Verification items for the finished model (mm, model axes). Round coordinates to 2 decimals unless told otherwise and drop trailing zeros. Write each loop counter-clockwise with the first axis right and the second up, starting at its lowest first coordinate (ties: lowest second). Pieces come first, ordered by that corner, then holes. Notation, with made-up numbers: M 9,22 L 61,22 A22 ccw 61,34 Z; hole C 56.25,67.25 d3. An arc over 180 degrees is marked long. Answer in a Markdown table with one row per item. Add a question column.
1. Sectioned sample at B-B on x = 18.5. Record the cut outline in (y, z) (3 decimals), plus the area to 3 significant figures.
2. Sectioned sample at D-D on z = -62.5. Record the cut outline in (x, y) (3 decimals).
3. Sectioned sample at C-C on x = 30. Record the cut outline in (y, z) (3 decimals).
4. Go/stop test with flat-tipped pins: pin 1 Ø3.5 at (x, z) = (37.11, -55.54) entering from +Y; pin 2 Ø1.9 at (y, z) = (-1.5, -24.5) entering from -X; pin 3 Ø2 at (x, y) = (4.5, 2) entering from -Z; pin 4 Ø4 at (x, z) = (65.52, 13.03) entering from -Y (3 decimals). Record where each tip stops, or that it passes through.
5. Sectioned sample at A-A on z = -3.5. Record the cut outline in (x, y) (3 decimals).
6. Material ranges on probe 1 along Y at (x, z) = (0, -70) (3 decimals); probe 2 along Z at (x, y) = (44.5, 0); probe 3 along Z at (x, y) = (42, 2.25), recorded low to high.
```python
from build123d import *

# Parameters (mm, degrees)
SKETCH1_R                                       = 7.5
BOSS_EXTRUDE1_DEPTH                             = 3.175
CIRPATTERN1_COUNT                               = 3
CIRPATTERN1_ANGLE                               = 135
M3_CLEARANCE_HOLE1_D                            = 3.2
M3_CLEARANCE_HOLE1_DEPTH                        = 15
CSK_FOR_M3_FLAT_HEAD_MACHINE_SCREW1_D           = 3.2
CSK_FOR_M3_FLAT_HEAD_MACHINE_SCREW1_CSINK_D     = 6.3
CSK_FOR_M3_FLAT_HEAD_MACHINE_SCREW1_CSINK_ANGLE = 90
CUT_EXTRUDE1_REACH                              = 107.268
FILLET1_R                                       = 3.175
CUT_EXTRUDE2_REACH                              = 107.268
SKETCH11_W                                      = 9.65
SKETCH11_H                                      = 32.732103654
F_1_4_CLEARANCE_HOLE1_D                         = 6.7564


with BuildPart() as part:
    # Sketch1 → Boss-Extrude1 (new, symmetric)
    with BuildSketch(Plane(origin=(0, 0, 0), x_dir=(1, 0, 0), z_dir=(0, 1, 0))):
        with BuildLine():
            Line((-13.85, 35), (-7.5, 35))
            Line((-7.5, 35), (-7.5, 15))
            Line((-7.5, 15), (-16.770509831, 15))
            ThreePointArc((-16.770509831, 15), (-18.002512666, -13.496649128), (9.696699141, -20.303300859))
            Line((9.696699141, -20.303300859), (46.966384428, -57.572986146))
            ThreePointArc((46.966384428, -57.572986146), (68.644249266, 28.433379025), (-7.5, 73.920497834))
            Line((-7.5, 73.920497834), (-7.5, 45))
            Line((-7.5, 45), (-13.85, 45))
            Line((-13.85, 45), (-13.85, 35))
        make_face()
        with Locations(Location((0, 0, 0), (0, 0, 270))):
            Circle(SKETCH1_R, mode=Mode.SUBTRACT)
        with BuildLine():
            Line((20.303300859, -9.696699141), (46.898012061, -36.291410343))
            ThreePointArc((46.898012061, -36.291410343), (58.160567128, -11.568856096), (57.216234934, 15.581798996))
            Line((57.216234934, 15.581798996), (22.468570216, 1.188845008))
            ThreePointArc((22.468570216, 1.188845008), (22.067668809, -4.389532245), (20.303300859, -9.696699141))
        make_face(mode=Mode.SUBTRACT)
        with BuildLine():
            Line((7.5, 15), (7.5, 35))
            Line((7.5, 35), (13.85, 35))
            Line((13.85, 35), (13.85, 45))
            Line((13.85, 45), (7.5, 45))
            Line((7.5, 45), (7.5, 58.823804705))
            ThreePointArc((7.5, 58.823804705), (32.945314818, 49.30614801), (51.475983449, 29.439991983))
            Line((51.475983449, 29.439991983), (16.72831873, 15.047037996))
            Line((16.72831873, 15.047037996), (16.614758962, 15))
            Line((16.614758962, 15), (7.5, 15))
        make_face(mode=Mode.SUBTRACT)
    extrude(amount=BOSS_EXTRUDE1_DEPTH, both=True)

    # Sketch5 → M2.2x0.45 Tapped Hole1 (revolve, cut)
    with BuildSketch(Plane(origin=(0, 0, -74.3), x_dir=(0, 1, 0), z_dir=(1, 0, 0))):
        Polygon((0, 0), (0, 10.525753042), (0.875, 10), (0.875, 0), align=None)
    m2_2x0_45_tapped_hole1 = revolve(axis=Axis((0, 0, -80.65), (0, 0, 1)), mode=Mode.SUBTRACT)

    # CirPattern1: M2.2x0.45 Tapped Hole1 ×3 about axis
    cirpattern1_axis = Axis((0, 3.175, 0), (0, -1, 0))
    for i in range(1, CIRPATTERN1_COUNT):
        add(m2_2x0_45_tapped_hole1.rotate(cirpattern1_axis, i * CIRPATTERN1_ANGLE / (CIRPATTERN1_COUNT - 1)), mode=Mode.SUBTRACT)

    # M3 Clearance Hole1
    with Locations(Plane.ZY.offset(7.5)):
        with Locations((-25, 0)):
            Hole(M3_CLEARANCE_HOLE1_D / 2, depth=M3_CLEARANCE_HOLE1_DEPTH)

    # CSK for M3 Flat Head Machine Screw1 (through all)
    with Locations(Plane(origin=(0, 3.175, 0), x_dir=(1, 0, 0), z_dir=(0, 1, 0))):
        with Locations((65.516456731, -13.032033511), (37.112091566, 55.542170102)):
            CounterSinkHole(CSK_FOR_M3_FLAT_HEAD_MACHINE_SCREW1_D / 2, CSK_FOR_M3_FLAT_HEAD_MACHINE_SCREW1_CSINK_D / 2, counter_sink_angle=CSK_FOR_M3_FLAT_HEAD_MACHINE_SCREW1_CSINK_ANGLE)

    # Sketch10 → Cut-Extrude1 (cut, up to next)
    with BuildSketch(Plane(origin=(0, 3.175, 0), x_dir=(1, 0, 0), z_dir=(0, 1, 0)), mode=Mode.PRIVATE) as cut_extrude1_sk1:
        with BuildLine():
            Line((-8.622532015, 15), (-9.74506403, 15))
            ThreePointArc((-9.74506403, 15), (-8.622532015, 14.535032015), (-7.5, 15))
            Line((-7.5, 15), (-8.622532015, 15))
        make_face()
    cut_extrude1_tool1 = extrude(cut_extrude1_sk1.sketch, amount=-CUT_EXTRUDE1_REACH, mode=Mode.PRIVATE) & part.part
    # Sketch10 → Cut-Extrude1 (cut, up to next)
    with BuildSketch(Plane(origin=(0, 3.175, 0), x_dir=(1, 0, 0), z_dir=(0, 1, 0)), mode=Mode.PRIVATE) as cut_extrude1_sk2:
        with BuildLine():
            ThreePointArc((-7.035032015, 16.122532015), (-7.155873257, 16.730041964), (-7.5, 17.24506403))
            Line((-7.5, 17.24506403), (-7.5, 16.122532015))
            Line((-7.5, 16.122532015), (-7.5, 15))
            ThreePointArc((-7.5, 15), (-7.155873257, 15.515022066), (-7.035032015, 16.122532015))
        make_face()
    cut_extrude1_tool2 = extrude(cut_extrude1_sk2.sketch, amount=-CUT_EXTRUDE1_REACH, mode=Mode.PRIVATE) & part.part
    # Sketch10 → Cut-Extrude1 (cut, up to next)
    with BuildSketch(Plane(origin=(0, 3.175, 0), x_dir=(1, 0, 0), z_dir=(0, 1, 0)), mode=Mode.PRIVATE) as cut_extrude1_sk3:
        with BuildLine():
            Line((8.622532015, 15), (7.5, 15))
            ThreePointArc((7.5, 15), (8.622532015, 14.535032015), (9.74506403, 15))
            Line((9.74506403, 15), (8.622532015, 15))
        make_face()
    cut_extrude1_tool3 = extrude(cut_extrude1_sk3.sketch, amount=-CUT_EXTRUDE1_REACH, mode=Mode.PRIVATE) & part.part
    # Sketch10 → Cut-Extrude1 (cut, up to next)
    with BuildSketch(Plane(origin=(0, 3.175, 0), x_dir=(1, 0, 0), z_dir=(0, 1, 0)), mode=Mode.PRIVATE) as cut_extrude1_sk4:
        with BuildLine():
            ThreePointArc((7.5, 17.24506403), (7.035032015, 16.122532015), (7.5, 15))
            Line((7.5, 15), (7.5, 16.122532015))
            Line((7.5, 16.122532015), (7.5, 17.24506403))
        make_face()
    cut_extrude1_tool4 = extrude(cut_extrude1_sk4.sketch, amount=-CUT_EXTRUDE1_REACH, mode=Mode.PRIVATE) & part.part
    # Sketch10 → Cut-Extrude1 (cut, up to next)
    with BuildSketch(Plane(origin=(0, 3.175, 0), x_dir=(1, 0, 0), z_dir=(0, 1, 0)), mode=Mode.PRIVATE) as cut_extrude1_sk5:
        with BuildLine():
            ThreePointArc((7.5, 35), (7.035032015, 33.877467985), (7.5, 32.75493597))
            Line((7.5, 32.75493597), (7.5, 33.877467985))
            Line((7.5, 33.877467985), (7.5, 35))
        make_face()
    cut_extrude1_tool5 = extrude(cut_extrude1_sk5.sketch, amount=-CUT_EXTRUDE1_REACH, mode=Mode.PRIVATE) & part.part
    # Sketch10 → Cut-Extrude1 (cut, up to next)
    with BuildSketch(Plane(origin=(0, 3.175, 0), x_dir=(1, 0, 0), z_dir=(0, 1, 0)), mode=Mode.PRIVATE) as cut_extrude1_sk6:
        with BuildLine():
            ThreePointArc((9.74506403, 35), (8.622532015, 35.464967985), (7.5, 35))
            Line((7.5, 35), (8.622532015, 35))
            Line((8.622532015, 35), (9.74506403, 35))
        make_face()
    cut_extrude1_tool6 = extrude(cut_extrude1_sk6.sketch, amount=-CUT_EXTRUDE1_REACH, mode=Mode.PRIVATE) & part.part
    # Sketch10 → Cut-Extrude1 (cut, up to next)
    with BuildSketch(Plane(origin=(0, 3.175, 0), x_dir=(1, 0, 0), z_dir=(0, 1, 0)), mode=Mode.PRIVATE) as cut_extrude1_sk7:
        with BuildLine():
            ThreePointArc((-7.035032015, 33.877467985), (-7.155873257, 34.484977934), (-7.5, 35))
            Line((-7.5, 35), (-7.5, 33.877467985))
            Line((-7.5, 33.877467985), (-7.5, 32.75493597))
            ThreePointArc((-7.5, 32.75493597), (-7.155873257, 33.269958036), (-7.035032015, 33.877467985))
        make_face()
    cut_extrude1_tool7 = extrude(cut_extrude1_sk7.sketch, amount=-CUT_EXTRUDE1_REACH, mode=Mode.PRIVATE) & part.part
    # Sketch10 → Cut-Extrude1 (cut, up to next)
    with BuildSketch(Plane(origin=(0, 3.175, 0), x_dir=(1, 0, 0), z_dir=(0, 1, 0)), mode=Mode.PRIVATE) as cut_extrude1_sk8:
        with BuildLine():
            Line((-8.622532015, 35), (-7.5, 35))
            ThreePointArc((-7.5, 35), (-8.622532015, 35.464967985), (-9.74506403, 35))
            Line((-9.74506403, 35), (-8.622532015, 35))
        make_face()
    cut_extrude1_tool8 = extrude(cut_extrude1_sk8.sketch, amount=-CUT_EXTRUDE1_REACH, mode=Mode.PRIVATE) & part.part
    add(cut_extrude1_tool1.solids().sort_by_distance((-8.622532, 3.175, -14.811461))[0], mode=Mode.SUBTRACT)
    add(cut_extrude1_tool2.solids().sort_by_distance((-7.311461, 3.175, -16.122532))[0], mode=Mode.SUBTRACT)
    add(cut_extrude1_tool3.solids().sort_by_distance((8.622532, 3.175, -14.811461))[0], mode=Mode.SUBTRACT)
    add(cut_extrude1_tool4.solids().sort_by_distance((7.311461, 3.175, -16.122532))[0], mode=Mode.SUBTRACT)
    add(cut_extrude1_tool5.solids().sort_by_distance((7.311461, 3.175, -33.877468))[0], mode=Mode.SUBTRACT)
    add(cut_extrude1_tool6.solids().sort_by_distance((8.622532, 3.175, -35.188539))[0], mode=Mode.SUBTRACT)
    add(cut_extrude1_tool7.solids().sort_by_distance((-7.311461, 3.175, -33.877468))[0], mode=Mode.SUBTRACT)
    add(cut_extrude1_tool8.solids().sort_by_distance((-8.622532, 3.175, -35.188539))[0], mode=Mode.SUBTRACT)

    # Fillet1
    fillet1_edges = [part.edges().sort_by_distance(p)[0] for p in [
        (-7.5, 0, -45),
        (9.696699141, 0, 20.303300859),
        (7.5, 0, -58.823804705),
        (7.5, 0, -45),
        (16.614758962, 0, -15),
        (51.475983449, 0, -29.439991983),
        (46.898012061, 0, 36.291410343),
        (57.216234934, 0, -15.581798996),
        (22.468570216, 0, -1.188845008),
        (20.303300859, 0, 9.696699141),
    ]]
    fillet(fillet1_edges, radius=FILLET1_R)

    # Sketch11 → Cut-Extrude2 (cut, up to next)
    with BuildSketch(Plane(origin=(0, 3.175, 0), x_dir=(1, 0, 0), z_dir=(0, 1, 0)), mode=Mode.PRIVATE) as cut_extrude2_sk1:
        with Locations((-18.675, -1.366051827)):
            Rectangle(SKETCH11_W, SKETCH11_H)
    cut_extrude2_tool1 = extrude(cut_extrude2_sk1.sketch, amount=-CUT_EXTRUDE2_REACH, mode=Mode.PRIVATE) & part.part
    add(cut_extrude2_tool1.solids().sort_by_distance((-18.675, 3.175, 1.366052))[0], mode=Mode.SUBTRACT)

    # 1/4 Clearance Hole1 (through all)
    with Locations(Plane(origin=(0, 3.175, 0), x_dir=(1, 0, 0), z_dir=(0, 1, 0))):
        with Locations((60.541360174, -28.230899884)):
            Hole(F_1_4_CLEARANCE_HOLE1_D / 2)


solid = part.part
```
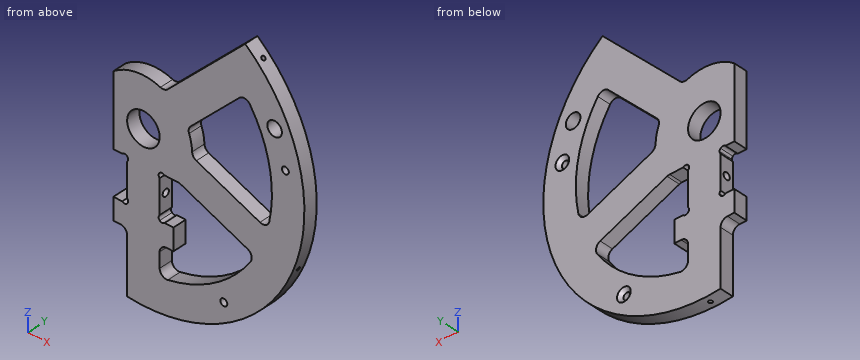
Geometry check:
| question | item | result |
|---|---|---|
| 1 | outline | M -3.175,-71.96 L 3.175,-71.96 L 3.175,-56.34 L -3.175,-56.34 Z; M -3.175,-15.781 L 3.175,-15.781 L 3.175,29.107 L -3.175,29.107 Z |
| 1 | area | 384 mm2 |
| 2 | outline | M -7.5,-3.175 L 40.178,-3.175 L 40.178,3.175 L -7.5,3.175 Z |
| 3 | outline | M -3.175,-67.974 L 3.175,-67.974 L 3.175,-51.152 L -3.175,-51.152 Z; M -3.175,-20.544 L 3.175,-20.544 L 3.175,-4.308 L -3.175,-4.308 Z; M -3.175,19.393 L 3.175,19.393 L 3.175,40.607 L -3.175,40.607 Z |
| 4 | pin 1 | stops at y = 1.78 |
| 4 | pin 2 | stops at x = -7.5 |
| 4 | pin 3 | stops at z = -74.22 |
| 4 | pin 4 | stops at y = -3.175 |
| 5 | outline | M -13.85,-3.175 L -6.633,-3.175 L -6.633,3.175 L -13.85,3.175 Z; M 6.633,-3.175 L 28.048,-3.175 L 28.048,3.175 L 6.633,3.175 Z; M 59.197,-3.175 L 74.218,-3.175 L 74.218,3.175 L 59.197,3.175 Z |
| 6 | probe 1 | y = -3.175 to -0.875, 0.875 to 3.175 |
| 6 | probe 2 | z = -59.5 to -39.19, -26.55 to -10.31, 33.87 to 55.11 |
| 6 | probe 3 | z = -61.29 to -41.86, -25.51 to -9.28, 31.39 to 52.61 |
